Read the model definition and answer for the solid it produces. Units are mm, in the model's axes. A direction names the side the tool comes from. Coordinates: 2 decimals unless noted, no trailing zeros. Order: outer loops, then holes, each group sorted by start corner. A loop starts at its lowest first (then second) coordinate and runs counter-clockwise, first axis right, second up. Notation, with made-up numbers: (33, 30.25) - (40, 30.25) arc R23 ccw to (40, 48.25) - close; hole circle Ø9 at (-20.75, 77.5). An arc over 180 degrees is marked (long way). Use one line per item in the form item = value. Start each with the question number.
from build123d import *

# Parameters (mm, degrees)
EXTRUDE_2_DEPTH     = 30
EXTRUDE_START       = -20
EXTRUDE_1_DEPTH     = 20
CUT_EXTRUDE_1_REACH = 59.671


# Read off the part's stored shape, not the designer's step: 拉伸-薄壁1
with BuildPart() as part:
    # 草图1 → 凸台-拉伸2 (new, symmetric)
    with BuildSketch(Plane.XY):
        Polygon((-26, 5), (26, 5), (26, -5), (10, -5), (12.886751346, 0), (-12.886751346, 0), (-10, -5), (-26, -5), align=None)
    extrude(amount=EXTRUDE_2_DEPTH, both=True)

    # 拉伸-薄壁1 outline → 拉伸-薄壁1 (add)
    with BuildSketch(Plane(origin=(26, 0, 0), x_dir=(0, 0, -1), z_dir=(1, 0, 0)).offset(EXTRUDE_START)):
        with BuildLine():
            Line((15, 5), (15, 23))
            ThreePointArc((15, 23), (0, 38), (-15, 23))
            Line((-15, 23), (-15, 5))
            Line((-15, 5), (15, 5))
        make_face()
        with BuildLine():
            ThreePointArc((-10, 23), (0, 33), (10, 23))
            Line((10, 23), (10, 10))
            Line((10, 10), (-10, 10))
            Line((-10, 10), (-10, 23))
        make_face(mode=Mode.SUBTRACT)
    extrude(amount=EXTRUDE_1_DEPTH)

    # 草图6 → 切除-拉伸1 (cut, up to next)
    with BuildSketch(Plane(origin=(0, 20, 15), x_dir=(1, 0, 0), z_dir=(0, 0, 1)), mode=Mode.PRIVATE) as cut_extrude_1_sk1:
        Polygon((22.5, -2.607695155), (16.5, 0.856406461), (10.5, -2.607695155), (10.5, -9.535898385), (16.5, -13), (22.5, -9.535898385), align=None)
    cut_extrude_1_tool1 = extrude(cut_extrude_1_sk1.sketch, amount=-CUT_EXTRUDE_1_REACH, mode=Mode.PRIVATE) & part.part
    add(cut_extrude_1_tool1.solids().sort_by_distance((16.5, 13.928203, 15))[0], mode=Mode.SUBTRACT)


solid = part.part
Q1. A cutting plane is placed at D-D (x = -21). Give the vertices of the cut face in (y, z), then the cut area to 3 significant figures.
Q2. A cutting plane is placed at C-C (z = 19.5). Give the vertices of the cut face in (x, y).
Q3. A cutting plane is placed at A-A (y = 14). Give the vertices of the cut face in (x, z).
Q4. A cutting plane is placed at B-B (z = -6). Give the vertices of the cut face in (x, y), then the cut area to 3 significant figures.
Q5. Which of the six approach directions +Z, -Z, +X, -X, +Y, -Y give full straight-line access (tool end or side, diameter ignored) to faces 5 (the cylindrical face through (16, 38, 0)), 6 (the cylindrical face through (16, 33, 0)), 7 (the flat face through (10.5, 14, 13)), 8 (the flat face through (18, -5, 0)), 9 (the flat face through (6, 21.7, 10.2))?
Q6. Consider probe 1 along Z at (x, y) = (23.5, 19.5); probe 2 along Y at (x, z) = (12.5, 2); probe 3 along Y at (x, z) = (-23.5, -25). Determine where each line is inside the solid, lowest interval first.
Q7. Given P1, Ø1.3, axis at x = 23, z = 2, coming from the +Y side; P2, Ø1.5, axis at y = 13, z = 11.5, coming from the -X side; P3, Ø5, axis at x = -14.5, z = 17.5, coming from the +Y side, each flat-ended and moving along its own axis, determine where each tip first touches the part or whether it passes through.
Q8. For a pull along Y with two mould halves and no side action, classify faces 1 (the flat face through (-11.46, -2.47, 0.42)), 2 (the flat face through (13.458, 8.756, 0.21)), 3 (the flat face through (-26, 0, 0)), 4 (the flat face through (-18, -5, 0)) as +Y half, -Y half, draft (parallel to the pull), parting line (faces both ways), or undercut.
Result sheet:
q1.outline = (-5, -30) - (5, -30) - (5, 30) - (-5, 30) - close
q1.area = 600 mm^2
q2.outline = (-26, -5) - (-10, -5) - (-12.89, 0) - (12.89, 0) - (10, -5) - (26, -5) - (26, 5) - (-26, 5) - close
q3.outline = (6, -15) - (10.5, -15) - (10.5, -10) - (6, -10) - close; (6, 10) - (10.5, 10) - (10.5, 15) - (6, 15) - close; (22.5, -15) - (26, -15) - (26, -10) - (22.5, -10) - close; (22.5, 10) - (26, 10) - (26, 15) - (22.5, 15) - close
q4.outline = (-26, -5) - (-10, -5) - (-12.89, 0) - (12.89, 0) - (10, -5) - (26, -5) - (26, 10) - (21.7, 10) - (16.5, 7) - (11.3, 10) - (6, 10) - (6, 5) - (-26, 5) - close; (6, 31) - (26, 31) - (26, 36.75) - (6, 36.75) - close
q4.area = 605 mm^2
q5.face_5 = +X, -X, +Y
q5.face_6 = +X, -X
q5.face_7 = +Z, -Z
q5.face_8 = +Z, -Z, +X, -X, -Y
q5.face_9 = +Z, -Z, -X, +Y
q6.probe_1 = -15 to -10, 10 to 15
q6.probe_2 = -5 to -0.67, 0 to 9.31, 32.8 to 37.87
q6.probe_3 = -5 to 5
q7.P1 = 37.94
q7.P2 = 6
q7.P3 = 5
q8.face_1 = undercut
q8.face_2 = undercut
q8.face_3 = draft
q8.face_4 = -Y half
